```python
from build123d import *

# Parameters (mm, degrees)
F1_DEPTH = 76.2
F2_R     = 1.26999


# Not quite as in the source:
# - a fillet or chamfer is up to 0.001 mm smaller than in the source, because OpenCascade refuses the exact size


with BuildPart() as f1:
    # F0 (on Front) → F1 (new body)
    with BuildSketch(Plane.XZ):
        with BuildLine():
            Line((-22.225, 19.05), (-24.765, 19.05))
            Line((-24.765, 19.05), (-24.765, -30.1625))
            Line((-24.765, -30.1625), (0, -30.1625))
            Line((0, -30.1625), (0, -25.4))
            Line((0, -25.4), (-21.43125, -25.4))
            ThreePointArc((-21.43125, -25.4), (-22.7862660076, -25.9612660076), (-22.225, -24.60625))
            Line((-22.225, -24.60625), (-22.225, 19.05))
        make_face()
        with BuildLine():
            Line((0, -25.4), (0, -30.1625))
            Line((0, -30.1625), (24.765, -30.1625))
            Line((24.765, -30.1625), (24.765, 19.05))
            Line((24.765, 19.05), (22.225, 19.05))
            Line((22.225, 19.05), (22.225, -24.60625))
            ThreePointArc((22.225, -24.60625), (22.7862660076, -24.8387339924), (23.01875, -25.4))
            ThreePointArc((23.01875, -25.4), (22.225, -26.19375), (21.43125, -25.4))
            Line((21.43125, -25.4), (0, -25.4))
        make_face()
    extrude(amount=F1_DEPTH)

    # F2 (radius 1.27 in the source; OpenCascade refuses exactly that, so slightly less here)
    f2_edges = [f1.edges().sort_by_distance(p)[0] for p in [
        (24.765, -38.1, 19.05),
        (22.225, -38.1, 19.05),
        (23.495, 0, 19.05),
        (23.495, -76.2, 19.05),
        (-22.225, -38.1, 19.05),
        (-24.765, -38.1, 19.05),
        (-23.495, 0, 19.05),
        (-23.495, -76.2, 19.05),
        (-24.765, -76.2, -5.55625),
        (24.765, -76.2, -5.55625),
        (24.765, 0, -5.55625),
        (-24.765, 0, -5.55625),
        (-24.765, -38.1, -30.1625),
        (24.765, -38.1, -30.1625),
        (0, 0, -30.1625),
        (0, -76.2, -30.1625),
    ]]
    fillet(f2_edges, radius=F2_R)


solid = f1.part
```
For this review, take the finished solid that the model builds, in its own axes (mm). A direction names the side the tool comes from. Coordinates: 2 decimals unless noted, no trailing zeros. Write each loop counter-clockwise with the first axis right and the second up, starting at its lowest first coordinate (ties: lowest second). Pieces come first, ordered by that corner, then holes.
(1) For pin 1 Ø3 at (x, y) = (17.5, -15.5) entering from +Z; pin 2 Ø2.5 at (x, z) = (-22.225, -25.4) entering from +Y, all flat-tipped, find the tip position at first contact; note any pin that passes through.
(2) Tool access review of faces 4 (the face through (-22.225, -38, -4)), 5 (the face through (0, -76.2, -26)): name each direction out of +Z, -Z, +X, -X, +Y, -Y from which nothing blocks a thin tool from reaching the whole face with its end or side.
(3) Add section C-C on x = 3. Give the boundary of the cut face in (y, z), then the cut area to 3 significant figures.
(4) The part is to be moulded in two halves that separate along X. For faces 1 (the face through (-22.767, -37.567, -25.979)), 2 (the face through (-24.765, -38, -5)), 3 (the face through (0, 0, -26)), say which applies: +X half, -X half, draft (parallel to the pull), parting line (faces both ways), or undercut.
(5) Add section A-A on z = 3.5. Give the boundary of the cut face in (x, y) (3 decimals).
(6) Wall thickness on probe 1 along X at (y, z) = (-70, -8) (3 decimals); probe 2 along Z at (x, y) = (6, -19.5); probe 3 along X at (y, z) = (-38, -25) (3 decimals): over which ranges is each line inside the solid? List them lowest first.
Answer sheet:
1. pin 1: stops at z = -25.4
1. pin 2: stops at y = 0
2. face 4: +Z, +Y, -Y
2. face 5: +Z, -Z, +X, -X, -Y
3. outline: (-76.2, -28.89) arc R1.27 ccw to (-74.93, -30.16) - (-1.27, -30.16) arc R1.27 ccw to (0, -28.89) - (0, -25.4) - (-76.2, -25.4) - close
3. area: 362 mm2
4. face 1: undercut
4. face 2: -X half
4. face 3: draft
5. outline: (-24.765, -74.93) arc R1.27 ccw to (-23.495, -76.2) - (-22.225, -76.2) - (-22.225, 0) - (-23.495, 0) arc R1.27 ccw to (-24.765, -1.27) - close; (22.225, -76.2) - (23.495, -76.2) arc R1.27 ccw to (24.765, -74.93) - (24.765, -1.27) arc R1.27 ccw to (23.495, 0) - (22.225, 0) - close
6. probe 1: x = -24.765 to -22.225, 22.225 to 24.765
6. probe 2: z = -30.16 to -25.4
6. probe 3: x = -24.765 to -22.911, 22.911 to 24.765
